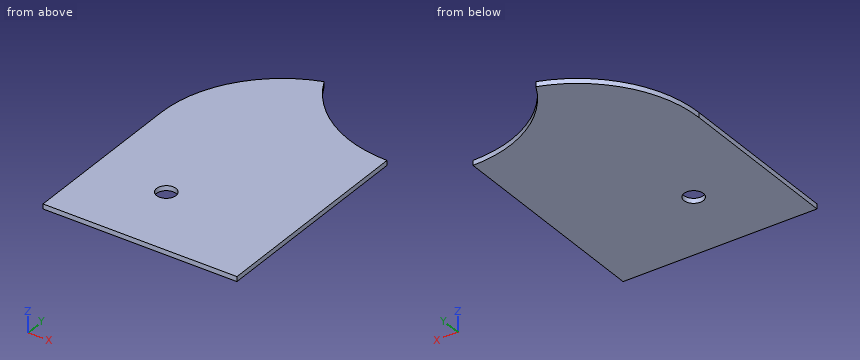
```python
from build123d import *

# Parameters (mm, degrees)
CYLINDER016_R     = 51
CYLINDER016_DEPTH = 10
CYLINDER_R        = 4
CYLINDER_DEPTH    = 10
BOX_W             = 80
BOX_H             = 120
BOX_DEPTH         = 2
FILLET_R          = 50


with BuildPart() as cylinder017:
    # Cylinder016 → Cylinder016 (new body)
    with BuildSketch(Plane.XY):
        Circle(CYLINDER016_R)
    extrude(amount=CYLINDER016_DEPTH)


with BuildPart() as cylinder:
    # Cylinder → Cylinder (new body)
    with BuildSketch(Plane(origin=(50, -110, 0), x_dir=(1, 0, 0), z_dir=(0, 0, 1))):
        Circle(CYLINDER_R)
    extrude(amount=CYLINDER_DEPTH)


with BuildPart() as cut010:
    # Box → Box (new body)
    with BuildSketch(Plane(origin=(0, -140, 0), x_dir=(1, 0, 0), z_dir=(0, 0, 1))):
        with Locations((40, 60)):
            Rectangle(BOX_W, BOX_H)
    extrude(amount=BOX_DEPTH)

    # Fillet
    fillet_edges = [cut010.edges().sort_by_distance(p)[0] for p in [
        (80, -20, 1),
    ]]
    fillet(fillet_edges, radius=FILLET_R)

    # Cut: cut Cylinder
    add(cylinder.part, mode=Mode.SUBTRACT)

    # Cut010: cut Cylinder017
    add(cylinder017.part, mode=Mode.SUBTRACT)


with BuildPart() as part_mirroring:
    # Part__Mirroring: instance of Cut010
    add(cut010.part.mirror(Plane(origin=(0, 0, 0), x_dir=(0, -1, 0), z_dir=(1, 0, 0))))


solid = part_mirroring.part
```
Read the model definition and answer for the solid it produces. Units are mm, in the model's axes. Coordinates: 2 decimals unless noted, no trailing zeros. Write each loop counter-clockwise with the first axis right and the second up, starting at its lowest first coordinate (ties: lowest second). Pieces come first, ordered by that corner, then holes. Notation, with made-up numbers: (-14, -32) -> (-10, -32) arc R21 cw to (-10, 5) -> close; hole circle Ø7 at (59.5, 47). An arc over 180 degrees is marked (long way). Return JSON: item names as keys, results as strings.
1. Find the intervals of material crossed by line 1 along X through (y, z) = (-110, 1.6); line 2 along X through (y, z) = (-113.5, 0.85); line 3 along Y through (x, z) = (-47, 0.5), in increasing order. Write a range as from..to.
Found:
{"line 1": "-80..-54, -46..0", "line 2": "-80..-51.94, -48.06..0", "line 3": "-140..-112.65, -107.35..-22.98"}
2. A cutting plane is placed at C-C (x = -51). Determine the outline of the cut face in (y, z).
Found:
{"outline": "(-140, 0) -> (-113.87, 0) -> (-113.87, 2) -> (-140, 2) -> close; (-106.13, 0) -> (-24.62, 0) -> (-24.62, 2) -> (-106.13, 2) -> close"}
3. A cutting plane is placed at B-B (z = 0.9). Determine the outline of the cut face in (x, y).
Found:
{"outline": "(-80, -140) -> (0, -140) -> (0, -51) arc R51 cw to (-45.75, -22.54) arc R50 ccw to (-80, -70) -> close; hole circle Ø8 at (-50, -110)"}
4. A cutting plane is placed at D-D (x = -70.5). Determine the outline of the cut face in (y, z), and give its area (3 significant figures).
Found:
{"outline": "(-140, 0) -> (-40.68, 0) -> (-40.68, 2) -> (-140, 2) -> close", "area": "199 mm2"}
5. A cutting plane is placed at A-A (y = -110). Determine the outline of the cut face in (x, z).
Found:
{"outline": "(-80, 0) -> (-54, 0) -> (-54, 2) -> (-80, 2) -> close; (-46, 0) -> (0, 0) -> (0, 2) -> (-46, 2) -> close"}
